Check sheet for the modelled part. Datum: model origin and axes. Units: mm. A direction names the side the tool comes from. Give positions to 0.01 mm unless a question says otherwise; leave off trailing zeros. Write each loop counter-clockwise with the first axis right and the second up, starting at its lowest first coordinate (ties: lowest second). Pieces come first, ordered by that corner, then holes. Notation, with made-up numbers: M 36,56.25 L 95,56.25 A14 cw 95,63.25 Z; hole C 4,3 d4. An arc over 180 degrees is marked long. Write item = value, one per line. Start each with the question number.
1) Mould release check, pull along X, two halves, no side actions. Record for faces 1 (the flat face through (29.3, 12, -6)), 2 (the flat face through (54, 20, -17)), 3 (the cylindrical face through (70.307, 10.533, -2.028)), 4 (the cylindrical face through (22, 10, -5)): released by +X, released by -X, zero draft, split by the parting line, or undercut.
2) Scan lines: line 1 along Y through (x, z) = (12, -1.05) (3 decimals); line 2 along X through (y, z) = (7.5, -2.25); line 3 along Z through (x, y) = (11.5, 3.5). Record each from-to range of solid material in increasing order. Write a range as [from, to].
3) Access from +Z, -Z, +X, -X, +Y, -Y to the whole of each face (thin tool, end or side, straight path). Record for faces 5 (the flat face through (60, 10, -11)), 6 (the flat face through (41, 3, 0)), 7 (the flat face through (54.7, 12, -6)).
4) Cross-section at D-D, the plane x = 42. Record the cut outline in (y, z), plus the area to 3 significant figures.
5) Cross-section at A-A, the plane y = 10. Record the cut outline in (x, z) (3 decimals), plus the area to 3 significant figures.
6) Cross-section at C-C, the plane z = -23.25. Record the cut outline in (x, y).
7) Go/stop test with flat-tipped pins: pin 1 (6 mm diameter, centred on y = 11.5, z = -22.5, fed in from -X); pin 2 (1 mm diameter, centred on y = 15, z = -16.5, fed in from +X); pin 3 (2 mm diameter, centred on y = 14.5, z = -14.5, fed in from +X). Record where each tip stops, or that it passes through.
8) Cross-section at B-B, the plane x = 72. Record the cut outline in (y, z) (3 decimals).
```python
from build123d import *

# Parameters (mm, degrees)
BOSS_EXTRUDE1_DEPTH = 20
SKETCH2_R           = 1.775
CUT_EXTRUDE1_DEPTH  = 5
FILLET1_R           = 3
FILLET2_R           = 5
BOSS_EXTRUDE2_DEPTH = 4


with BuildPart() as part:
    # Sketch1 → Boss-Extrude1 (new body)
    with BuildSketch(Plane(origin=(0, 0, 0), x_dir=(1, 0, 0), z_dir=(0, 1, 0))):
        with BuildLine():
            Line((0, 0), (0, 4))
            Line((0, 4), (24, 4))
            Line((24, 4), (24, 12))
            ThreePointArc((24, 12), (42, 30), (60, 12))
            Line((60, 12), (60, 4))
            Line((60, 4), (84, 4))
            Line((84, 4), (84, 0))
            Line((84, 0), (54.7, 0))
            Line((54.7, 0), (54.7, 12))
            ThreePointArc((54.7, 12), (42, 24.7), (29.3, 12))
            Line((29.3, 12), (29.3, 0))
            Line((29.3, 0), (0, 0))
        make_face()
    extrude(amount=BOSS_EXTRUDE1_DEPTH)

    # Sketch2 → Cut-Extrude1 (cut, through all)
    with BuildSketch(Plane(origin=(0, 0, -4), x_dir=(-1, 0, 0), z_dir=(0, 0, -1))):
        with Locations((-72, 10)):
            Circle(SKETCH2_R)
        with Locations((-12, 10)):
            Circle(SKETCH2_R)
    extrude(amount=-CUT_EXTRUDE1_DEPTH, mode=Mode.SUBTRACT)

    # Fillet1
    fillet1_edges = [part.edges().sort_by_distance(p)[0] for p in [
        (0, 0, -2),
        (84, 0, -2),
        (84, 20, -2),
        (0, 20, -2),
    ]]
    fillet(fillet1_edges, radius=FILLET1_R)

    # Fillet2
    fillet2_edges = [part.edges().sort_by_distance(p)[0] for p in [
        (24, 10, -4),
        (60, 10, -4),
    ]]
    fillet(fillet2_edges, radius=FILLET2_R)

    # Sketch4 → Boss-Extrude2 (add)
    with BuildSketch(Plane.XZ):
        with BuildLine():
            Line((29.3, 0), (54.7, 0))
            Line((54.7, 0), (54.7, -12))
            ThreePointArc((54.7, -12), (42, -24.7), (29.3, -12))
            Line((29.3, -12), (29.3, 0))
        make_face()
    extrude(amount=-BOSS_EXTRUDE2_DEPTH)


solid = part.part
```
Reply:
q1.face_1 = undercut
q1.face_2 = zero draft
q1.face_3 = undercut
q1.face_4 = released by -X
q2.line_1 = [0, 8.225], [11.775, 20]
q2.line_2 = [0, 29.3], [54.7, 84]
q2.line_3 = [-4, 0]
q3.face_5 = -Z, +X, +Y, -Y
q3.face_6 = +Z, +X, -X, +Y, -Y
q3.face_7 = +Z, +Y
q4.outline = M 0,-30 L 20,-30 L 20,-24.7 L 4,-24.7 L 4,0 L 0,0 Z
q4.area = 205 mm2
q5.outline = M 0,-4 L 10.225,-4 L 10.225,0 L 0,0 Z; M 13.775,-4 L 19,-4 A5 cw 24,-9 L 24,-12 A18 ccw 60,-12 L 60,-9 A5 cw 65,-4 L 70.225,-4 L 70.225,0 L 54.7,0 L 54.7,-12 A12.7 cw 29.3,-12 L 29.3,0 L 13.775,0 Z; M 73.775,-4 L 84,-4 L 84,0 L 73.775,0 Z
q5.area = 557 mm2
q6.outline = M 27.95,0 L 56.05,0 L 56.05,20 L 47.89,20 L 47.89,4 L 36.11,4 L 36.11,20 L 27.95,20 Z
q7.pin_1 = 25.64
q7.pin_2 = 59.55
q7.pin_3 = 59.94
q8.outline = M 0,-4 L 8.225,-4 L 8.225,0 L 0,0 Z; M 11.775,-4 L 20,-4 L 20,0 L 11.775,0 Z
